```python
from build123d import *

# Parameters (mm, degrees)
BOSS_EXTRUDE1_DEPTH = 38.1
SKETCH2_R           = 12.7
CUT_EXTRUDE1_DEPTH  = 12.7


with BuildPart() as part:
    # Sketch1 → Boss-Extrude1 (new body)
    with BuildSketch(Plane(origin=(0, 0, 0), x_dir=(1, 0, 0), z_dir=(0, 1, 0))):
        with BuildLine():
            Line((-1003.209151546, 19.574124673), (-852.041766236, 170.741509982))
            Line((-852.041766236, 170.741509982), (-851.297817461, 171.485458758))
            ThreePointArc((-851.297817461, 171.485458758), (-827.400793586, 187.45293962), (-799.212331958, 193.059973256))
            Line((-799.212331958, 193.059973256), (-752.46588673, 193.059973256))
            Line((-752.46588673, 193.059973256), (636.970077719, 193.059973256))
            Line((636.970077719, 193.059973256), (682.664420499, 193.059973256))
            ThreePointArc((682.664420499, 193.059973256), (711.824898045, 187.259593633), (736.545957225, 170.741509982))
            Line((736.545957225, 170.741509982), (892.049393759, 15.238073448))
            ThreePointArc((892.049393759, 15.238073448), (914.624108082, -98.252679391), (818.411293566, -162.540026744))
            Line((818.411293566, -162.540026744), (812.279191118, -162.540026744))
            Line((812.279191118, -162.540026744), (-927.775000129, -162.540026744))
            Line((-927.775000129, -162.540026744), (-933.907102577, -162.540026744))
            ThreePointArc((-933.907102577, -162.540026744), (-1030.119917093, -98.252679391), (-1007.54520277, 15.238073448))
            Line((-1007.54520277, 15.238073448), (-1003.209151546, 19.574124673))
        make_face()
    extrude(amount=BOSS_EXTRUDE1_DEPTH)

    # Sketch2 → Cut-Extrude1 (cut)
    with BuildSketch(Plane.XZ):
        with Locations((-629.107102577, 58.400026744)):
            Circle(SKETCH2_R)
        with Locations((513.611293566, 58.400026744)):
            Circle(SKETCH2_R)
    extrude(amount=-CUT_EXTRUDE1_DEPTH, mode=Mode.SUBTRACT)


solid = part.part
```
Geometry check sheet. Reference: the model listing, model coordinates, mm. Round coordinates to 2 decimals unless told otherwise and drop trailing zeros. Loops run counter-clockwise (first coordinate to the right, second up) from the corner with the lowest first, then second, coordinate; pieces in that order, holes last. Notation, with made-up numbers: (-11.75, -12.75) - (47.25, -12.75) arc R28 cw to (47.25, 7.25) - close; hole circle Ø10 at (66.5, 29). An arc over 180 degrees is marked (long way). Use a Markdown table: item, result.
Q1. Material ranges on line 1 (X direction, y = 20, z = 61.5); line 2 (X direction, y = 24.5, z = 104); line 3 (Z direction, x = 817.5, y = 23.5), recorded low to high.
Solutions:
| item | result |
|---|---|
| line 1 | x = -1038 to 922.51 |
| line 2 | x = -1027.53 to 912.04 |
| line 3 | z = -89.79 to 162.54 |
Q2. Cross-section at A-A on y = 6.5. Record the cut outline in (x, z), plus the area to 3 significant figures.
Solutions:
| item | result |
|---|---|
| outline | (-1007.55, -15.24) - (-851.3, -171.49) arc R73.66 ccw to (-799.21, -193.06) - (682.66, -193.06) arc R76.2 ccw to (736.55, -170.74) - (892.05, -15.24) arc R104.14 ccw to (818.41, 162.54) - (-933.91, 162.54) arc R104.14 ccw to start; hole circle Ø25.4 at (-629.11, 58.4); hole circle Ø25.4 at (513.61, 58.4) |
| area | 647,000 mm2 |
Q3. Cross-section at B-B on z = -55. Record the cut outline in (x, y).
Solutions:
| item | result |
|---|---|
| outline | (-967.78, 0) - (852.29, 0) - (852.29, 38.1) - (-967.78, 38.1) - close |
Q4. Cross-section at C-C on x = -903. Record the cut outline in (y, z), plus the area to 3 significant figures.
Solutions:
| item | result |
|---|---|
| outline | (0, -119.78) - (38.1, -119.78) - (38.1, 162.54) - (0, 162.54) - close |
| area | 10,800 mm2 |
Q5. Go/stop test with flat-tipped pins: P1, Ø1, axis at y = 11, z = -90.5, coming from the -X side; P2, Ø4, axis at y = 17.5, z = 99, coming from the -X side; P3, Ø3, axis at y = 14.5, z = 1, coming from the -X side. Record where each tip stops, or that it passes through.
Solutions:
| item | result |
|---|---|
| P1 | stops at x = -932.78 |
| P2 | stops at x = -1030.63 |
| P3 | stops at x = -1021.77 |
